from build123d import *

# Parameters (mm, degrees)
F0_W     = 12.7
F0_H     = 63.5
F1_DEPTH = 50.8
F3_DEPTH = 12.7


# Not quite as in the source:
# - a pattern or mirror of a feature is missing from the dataset's text; its kind, count and spacing are read off the source's solid


with BuildPart() as f1:
    # F0 (on Right) → F1 (new body, symmetric)
    with BuildSketch(Plane.YZ):
        Rectangle(F0_W, F0_H)
    extrude(amount=F1_DEPTH, both=True)

    # F2 (on face) → F3 (cut)
    with BuildSketch(Plane(origin=(-50.8, 0, 0), x_dir=(0, -1, 0), z_dir=(-1, 0, 0))):
        Polygon((6.35, -22.225), (6.35, 22.225), (-6.35, 19.6872895852), (-6.35, -19.6872895852), align=None)
    f3 = extrude(amount=-F3_DEPTH, mode=Mode.SUBTRACT)

    # F3_copies: F3 across plane
    add(f3.mirror(Plane(origin=(0, 0, 0), x_dir=(0, 0, 1), z_dir=(1, 0, 0))), mode=Mode.SUBTRACT)


solid = f1.part
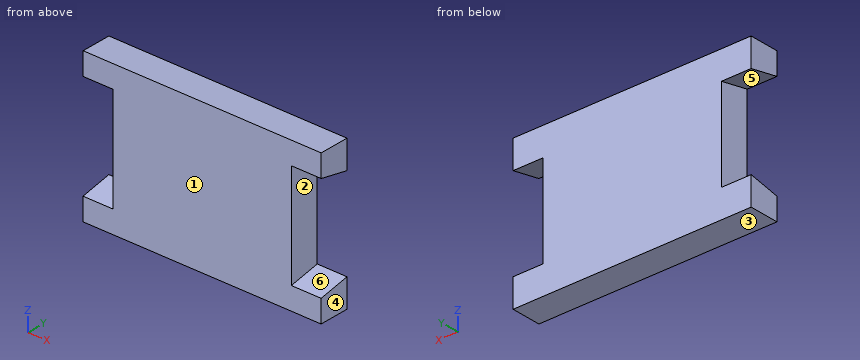
Input: part model. Units: mm. Frame: model coordinates. Face numbers are marked on the shaded views. A direction names the side the tool comes from. Round coordinates to 2 decimals unless told otherwise and drop trailing zeros. Order: outer loops, then holes, each group sorted by start corner. A loop starts at its lowest first (then second) coordinate and runs counter-clockwise, first axis right, second up. Notation, with made-up numbers: (-37.75, -30.75) - (-6.75, -30.75) arc R23 cw to (-6.75, -10.75) - close; hole circle Ø11 at (-31, 20). An arc over 180 degrees is marked (long way). Answer as a JSON object with one key per item and string values. Group by question number.
(1) Cut plane A-A (x = -44.5). Return loops of the section in (y, z) (3 decimals), then the cut area to 3 significant figures.
(2) Material intervals for probe 1 along X at (y, z) = (0.25, 2); probe 2 along Z at (x, y) = (-39, 1.5); probe 3 along Z at (x, y) = (44.5, 4), sorted ascending. Write a range as from..to.
(3) Cut plane B-B (y = 0.5). Return loops of the section in (x, z), then the cut area to 3 significant figures.
(4) Reachability of the marked faces 4, 5 and 6 from +Z, -Z, +X, -X, +Y, -Y: full face, straight path, thin tool, end or side. Return the list, or none.
(5) Draft query along Z for the marked faces 1, 2 and 3. Return one class per face: released by +Z, released by -Z, zero draft, split by the parting line, or undercut.
(6) Cut plane C-C (z = -15). Return loops of the section in (x, y), then the cut area to 3 significant figures.
(7) Cut plane D-D (y = 5.25). Return loops of the section in (x, z).
(8) Pin query (flat end, axial travel): P1, Ø2, axis at y = 3, z = -3.5, coming from the -X side; P2, Ø2, axis at x = 40.5, z = -1, coming from the -Y side. Return the tip coordinate at first contact, or that it passes through.
Here are the results:
{
 "1": {"outline": "(-6.35, -31.75) - (6.35, -31.75) - (6.35, -19.687) - (-6.35, -22.225) - close; (-6.35, 22.225) - (6.35, 19.687) - (6.35, 31.75) - (-6.35, 31.75) - close", "area": "274 mm^2"},
 "2": {"probe 1": "x = -38.1..38.1", "probe 2": "z = -31.75..-20.66, 20.66..31.75", "probe 3": "z = -31.75..-20.16, 20.16..31.75"},
 "3": {"outline": "(-50.8, -31.75) - (50.8, -31.75) - (50.8, -20.86) - (38.1, -20.86) - (38.1, 20.86) - (50.8, 20.86) - (50.8, 31.75) - (-50.8, 31.75) - (-50.8, 20.86) - (-38.1, 20.86) - (-38.1, -20.86) - (-50.8, -20.86) - close", "area": "5,390 mm^2"},
 "4": {"face 4": "+Z, -Z, +X, +Y, -Y", "face 5": "-X, -Y", "face 6": "+X, -Y"},
 "5": {"face 1": "zero draft", "face 2": "undercut", "face 3": "released by -Z"},
 "6": {"outline": "(-38.1, -6.35) - (38.1, -6.35) - (38.1, 6.35) - (-38.1, 6.35) - close", "area": "968 mm^2"},
 "7": {"outline": "(-50.8, -31.75) - (50.8, -31.75) - (50.8, -19.91) - (38.1, -19.91) - (38.1, 19.91) - (50.8, 19.91) - (50.8, 31.75) - (-50.8, 31.75) - (-50.8, 19.91) - (-38.1, 19.91) - (-38.1, -19.91) - (-50.8, -19.91) - close"},
 "8": {"P1": "stops at x = -38.1", "P2": "passes through"}
}
